```python
from build123d import *

# Parameters (mm, degrees)
BOSS_EXTRUDE2_DEPTH = 4
FILLET1_R           = 4
SKETCH6_R           = 1.5
CUT_EXTRUDE1_DEPTH  = 4
SKETCH3_R           = 1.5
CUT_EXTRUDE2_DEPTH  = 4


with BuildPart() as part:
    # Sketch2 → Boss-Extrude2 (new body)
    with BuildSketch(Plane.XY):
        Polygon((-87.081093968, -2.634474623), (-87.081093968, 16.923525377), (-46.695093968, 16.923525377), (-46.695093968, -2.634474623), (-39.075093968, -2.634474623), (-39.075093968, 32.365525377), (-67.081093968, 32.365525377), (-74.701093968, 32.365525377), (-159.701093968, 32.365525377), (-167.321093968, 32.365525377), (-215.327093968, 32.365525377), (-215.327093968, -2.634474623), (-207.707093968, -2.634474623), (-207.707093968, 16.923525377), (-167.321093968, 16.923525377), (-167.231910297, 16.736340115), (-167.321093968, 16.736752562), (-167.321093968, -2.634474623), (-159.701093968, -2.634474623), (-159.701093968, 16.923525377), (-94.701093968, 16.923525377), (-94.701093968, -2.634474623), align=None)
    extrude(amount=BOSS_EXTRUDE2_DEPTH)

    # Fillet1
    fillet1_edges = [part.edges().sort_by_distance(p)[0] for p in [
        (-39.075093968, 32.365525377, 2),
        (-39.075093968, -2.634474623, 2),
        (-94.701093968, -2.634474623, 2),
        (-159.701093968, -2.634474623, 2),
        (-215.327093968, -2.634474623, 2),
        (-215.327093968, 32.365525377, 2),
    ]]
    fillet(fillet1_edges, radius=FILLET1_R)

    # Sketch6 → Cut-Extrude1 (cut)
    with BuildSketch(Plane.XY.offset(4)):
        with Locations((-211.644093968, 12.224525377)):
            Circle(SKETCH6_R)
        with Locations((-163.384093968, 12.224525377)):
            Circle(SKETCH6_R)
        with Locations((-163.384093968, 2.064525377)):
            Circle(SKETCH6_R)
        with Locations((-211.644093968, 2.064525377)):
            Circle(SKETCH6_R)
        with Locations((-91.018093968, 12.224525377)):
            Circle(SKETCH6_R)
        with Locations((-42.758093968, 12.224525377)):
            Circle(SKETCH6_R)
        with Locations((-42.758093968, 2.064525377)):
            Circle(SKETCH6_R)
        with Locations((-91.018093968, 2.064525377)):
            Circle(SKETCH6_R)
    extrude(amount=-CUT_EXTRUDE1_DEPTH, mode=Mode.SUBTRACT)

    # Sketch3 → Cut-Extrude2 (cut)
    with BuildSketch(Plane.XY.offset(4)):
        with Locations((-145.701093968, 25.365525377)):
            Circle(SKETCH3_R)
        with Locations((-108.701093968, 25.365525377)):
            Circle(SKETCH3_R)
    extrude(amount=-CUT_EXTRUDE2_DEPTH, mode=Mode.SUBTRACT)


solid = part.part
```
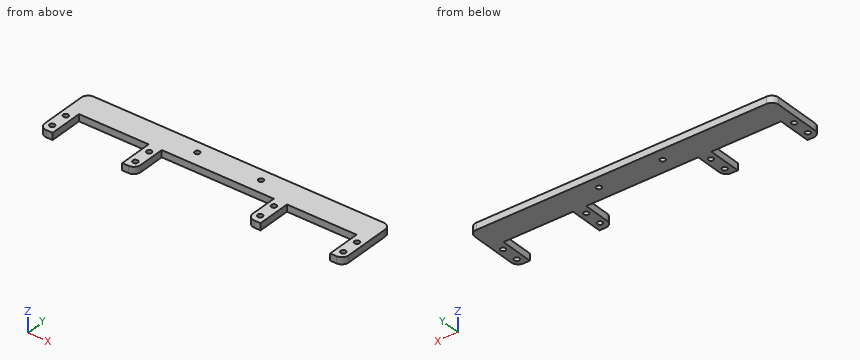
Design review of the part built by this model. Coordinates are the model's own, in mm. Coordinates: 2 decimals unless noted, no trailing zeros. Write each loop counter-clockwise with the first axis right and the second up, starting at its lowest first coordinate (ties: lowest second). Pieces come first, ordered by that corner, then holes.
1) Add section A-A (y = 8.5). Write out the cut boundary in (x, z), plus the area to 3 significant figures.
2) Insertion check: pin 1 (2.5 mm diameter, centred on x = -91.02, y = 2.06, fed in from -Z); pin 2 (5 mm diameter, centred on x = -163.38, y = 2.06, fed in from +Z); pin 3 (2 mm diameter, centred on x = -126.5, z = 2.5, fed in from -Y). Each pin has a flat end and moves straight along its axis. Give the tip position at first contact, or say it passes through.
3) To check wall thickness, follow L1, parallel to X at y = 16, z = 1.2; L2, parallel to X at y = 24.5, z = 1; L3, parallel to Y at x = -130, z = 3.7. State the ranges of each line that lie inside material, in increasing order.
4) Add section B-B (x = -179). Write out the cut boundary in (y, z), plus the area to 3 significant figures.
5) Add section C-C (z = 3.4). State how many separate pieces and enclosed holes the cut face has, plus the area to 3 significant figures.
Check result:
1. outline: (-215.33, 0) - (-207.71, 0) - (-207.71, 4) - (-215.33, 4) - close; (-167.32, 0) - (-159.7, 0) - (-159.7, 4) - (-167.32, 4) - close; (-94.7, 0) - (-87.08, 0) - (-87.08, 4) - (-94.7, 4) - close; (-46.7, 0) - (-39.08, 0) - (-39.08, 4) - (-46.7, 4) - close
1. area: 122 mm2
2. pin 1: passes through
2. pin 2: stops at z = 4
2. pin 3: stops at y = 16.92
3. L1: x = -215.33 to -207.71, -167.32 to -159.7, -94.7 to -87.08, -46.7 to -39.08
3. L2: x = -215.33 to -146.93, -144.48 to -109.93, -107.48 to -39.08
3. L3: y = 16.92 to 32.37
4. outline: (16.92, 0) - (32.37, 0) - (32.37, 4) - (16.92, 4) - close
4. area: 61.8 mm2
5. separate pieces: 1
5. enclosed holes: 10
5. area: 3,230 mm2
